```python
from build123d import *

# Parameters (mm, degrees)
CROQUIS1_W                   = 50
CROQUIS1_H                   = 50
SALIENTE_EXTRUIR1_DEPTH      = 5
SALIENTE_EXTRUIR2_REACH      = 65.295
SALIENTE_EXTRUIR2_END_RADIUS = 15
CROQUIS2_R                   = 7.5
CROQUIS4_R                   = 1.5
CORTAR_EXTRUIR1_DEPTH        = 5
REDONDEO1_R                  = 5
REDONDEO2_R                  = 5


with BuildPart() as part:
    # Croquis1 → Saliente-Extruir1 (new body)
    with BuildSketch(Plane.XY):
        Rectangle(CROQUIS1_W, CROQUIS1_H)
    extrude(amount=SALIENTE_EXTRUIR1_DEPTH)



with BuildPart() as body_2:
    # Croquis3 → Revolución1 (revolve)
    with BuildSketch(Plane(origin=(0, 0, -37.5), x_dir=(-1, 0, 0), z_dir=(0, 0, -1))):
        with BuildLine():
            Line((0, 15), (0, -15))
            ThreePointArc((0, -15), (15, 0), (0, 15))
        make_face()
    revolve(axis=Axis((0, 15, -37.5), (0, -1, 0)))


with BuildPart() as part_1:
    add(part.part)

    add(body_2.part)  # Saliente-Extruir2 merges body 2
    # Saliente-Extruir2: up to this sphere (the profile starts outside it)
    saliente_extruir2_end = Location((0, 0, -37.5)) * Sphere(SALIENTE_EXTRUIR2_END_RADIUS, mode=Mode.PRIVATE)
    # Croquis2 → Saliente-Extruir2 (add, up to the surface)
    with BuildSketch(Plane(origin=(0, 0, 0), x_dir=(-1, 0, 0), z_dir=(0, 0, -1)), mode=Mode.PRIVATE) as saliente_extruir2_sk1:
        with Locations(Location((0, 0, 0), (0, 0, 180))):
            Circle(CROQUIS2_R)
    saliente_extruir2_tool1 = extrude(saliente_extruir2_sk1.sketch, amount=SALIENTE_EXTRUIR2_REACH, mode=Mode.PRIVATE) - saliente_extruir2_end
    add(saliente_extruir2_tool1.solids().sort_by_distance((0, 0, 0))[0])

    # Croquis4 → Cortar-Extruir1 (cut)
    with BuildSketch(Plane(origin=(0, 0, 0), x_dir=(-1, 0, 0), z_dir=(0, 0, -1))):
        with Locations((-20, 20)):
            Circle(CROQUIS4_R)
        with Locations(Location((20, 20, 0), (0, 0, 180))):
            Circle(CROQUIS4_R)
        with Locations((20, -20)):
            Circle(CROQUIS4_R)
        with Locations(Location((-20, -20, 0), (0, 0, 180))):
            Circle(CROQUIS4_R)
    extrude(amount=-CORTAR_EXTRUIR1_DEPTH, mode=Mode.SUBTRACT)

    # Redondeo1
    redondeo1_edges = [part_1.edges().sort_by_distance(p)[0] for p in [
        (25, -25, 2.5),
        (-25, -25, 2.5),
        (-25, 25, 2.5),
        (25, 25, 2.5),
    ]]
    fillet(redondeo1_edges, radius=REDONDEO1_R)

    # Redondeo2
    redondeo2_edges = [part_1.edges().sort_by_distance(p)[0] for p in [
        (-7.5, 0, 0),
    ]]
    fillet(redondeo2_edges, radius=REDONDEO2_R)


solid = part_1.part
```
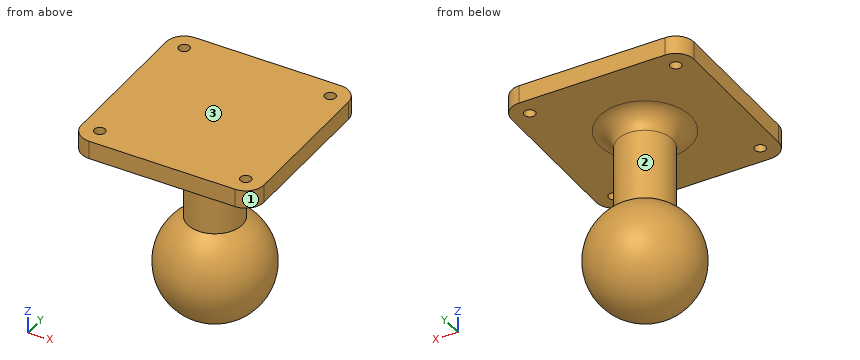
The model under review builds one solid part; all positions refer to its coordinate system, in mm. Face numbers are marked on the shaded views. Round coordinates to 2 decimals unless told otherwise and drop trailing zeros. Loops run counter-clockwise (first coordinate to the right, second up) from the corner with the lowest first, then second, coordinate; pieces in that order, holes last.
1) Clearance check with flat-ended pins moving along their axes: P1, Ø2.5, axis at x = -20, y = 20, coming from the +Z side; P2, Ø3.5, axis at x = 20, y = 20, coming from the -Z side; P3, Ø10, axis at y = 0, z = -12, coming from the +X side; P4, Ø1.5, axis at y = 10, z = -36.5, coming from the -X side. State where each tip first meets the part, or that it passes through.
Values follow:
P1: passes through
P2: stops at z = 0
P3: stops at x = 7.5
P4: stops at x = -11.77
2) The part is to be moulded in two halves that separate along Z. For the marked faces 1, 2 and 3, say which applies: pulls with the +Z half, pulls with the -Z half, needs draft (parallel to the pull), parting line crosses it, or undercut.
Values follow:
face 1: needs draft
face 2: undercut
face 3: pulls with the +Z half
3) Consider section A-A on y = 0. State the section outline as (x, z) points, then the cut area to 3 significant figures.
Values follow:
outline: (-25, 0) - (-12.5, 0) arc R5 cw to (-7.5, -5) - (-7.5, -24.51) arc R15 ccw (long way) to (7.5, -24.51) - (7.5, -5) arc R5 cw to (12.5, 0) - (25, 0) - (25, 5) - (-25, 5) - close
area: 1,310 mm2
4) Consider section B-B on z = -45. State the section outline as (x, y) points, then the cut area to 3 significant figures.
Values follow:
outline: circle Ø25.98 at (0, 0)
area: 530 mm2
5) Wall thickness on line 1 along Y through (x, z) = (-20, 2.6); line 2 along Z through (x, y) = (21.5, -13); line 3 along Z through (x, y) = (3.5, -8.5): over which ranges is each line inside the solid? List them lowest first.
Values follow:
line 1: y = -25 to -21.5, -18.5 to 18.5, 21.5 to 25
line 2: z = 0 to 5
line 3: z = -49.35 to -25.65, -1.25 to 5
